```python
from build123d import *

# Parameters (mm, degrees)
SKETCH1_W           = 218
SKETCH1_H           = 465
BOSS_EXTRUDE1_DEPTH = 2
SKETCH2_W           = 30
SKETCH2_H           = 20
CUT_EXTRUDE1_DEPTH  = 8
BOSS_EXTRUDE2_DEPTH = 2


with BuildPart() as part:
    # Sketch1 → Boss-Extrude1 (new body)
    with BuildSketch(Plane.XY):
        Rectangle(SKETCH1_W, SKETCH1_H)
    extrude(amount=BOSS_EXTRUDE1_DEPTH)

    # Sketch2 → Cut-Extrude1 (cut)
    with BuildSketch(Plane.XY.offset(2)):
        Polygon((-61, 190), (-91, 190), (-91, 180), (-91, 170), (-61, 170), align=None)
        Polygon((-61, 145), (-91, 145), (-91, 135), (-91, 125), (-61, 125), align=None)
        with Locations((-76, 90)):
            Rectangle(SKETCH2_W, SKETCH2_H)
        with Locations((-76, 45)):
            Rectangle(SKETCH2_W, SKETCH2_H)
        with Locations((-76, 0)):
            Rectangle(SKETCH2_W, SKETCH2_H)
        with Locations((-76, -45)):
            Rectangle(SKETCH2_W, SKETCH2_H)
        with Locations((-76, -90)):
            Rectangle(SKETCH2_W, SKETCH2_H)
        with Locations((-76, -135)):
            Rectangle(SKETCH2_W, SKETCH2_H)
        with Locations((-76, -180)):
            Rectangle(SKETCH2_W, SKETCH2_H)
    extrude(amount=-CUT_EXTRUDE1_DEPTH, mode=Mode.SUBTRACT)

    # Sketch3 → Boss-Extrude2 (add)
    with BuildSketch(Plane.XY.offset(2)):
        Polygon((111, 164.5), (109, 164.5), (109, 139.5), (109, 114.5), (111, 114.5), align=None)
        Polygon((111, 71.5), (109, 71.5), (109, 46.5), (109, 21.5), (111, 21.5), align=None)
        Polygon((111, -114.5), (109, -114.5), (109, -139.5), (109, -164.5), (111, -164.5), align=None)
        Polygon((111, -21.5), (109, -21.5), (109, -46.5), (109, -71.5), (111, -71.5), align=None)
    extrude(amount=-BOSS_EXTRUDE2_DEPTH)


solid = part.part
```
Geometry check sheet. Reference: the model listing, model coordinates, mm. Coordinates: 2 decimals unless noted, no trailing zeros. Order: outer loops, then holes, each group sorted by start corner. A loop starts at its lowest first (then second) coordinate and runs counter-clockwise, first axis right, second up.
Item 1: Section check B-B (z = 1.65). Count the separate pieces of the cut face and the enclosed holes in it, plus the area to 3 significant figures.
Item 2: Section check A-A (y = -180). Enter the section's corners in (x, z), plus the area to 3 significant figures.
Item 3: Scan lines: line 1 along X through (y, z) = (-171, 0.7); line 2 along X through (y, z) = (-77, 0.95). Record each from-to range of solid material in increasing order.
Item 4: Depth check by flat-ended pin: pin 1 (0.6 mm diameter, centred on y = 0, z = 1, fed in from +X); pin 2 (1 mm diameter, centred on x = 110.5, z = 0.5, fed in from -Y); pin 3 (0.6 mm diameter, centred on x = 110, z = 0.5, fed in from +Y); pin 4 (1 mm diameter, centred on x = -26.5, y = 151, fed in from -Z). Enter the tip coordinate at first touch or a pass-through.
Check sheet entries:
1. separate pieces: 1
1. enclosed holes: 9
1. area: 96,400 mm2
2. outline: (-109, 0) - (-91, 0) - (-91, 2) - (-109, 2) - close; (-61, 0) - (109, 0) - (109, 2) - (-61, 2) - close
2. area: 376 mm2
3. line 1: x = -109 to -91, -61 to 109
3. line 2: x = -109 to 109
4. pin 1: stops at x = 109
4. pin 2: stops at y = -164.5
4. pin 3: stops at y = 164.5
4. pin 4: stops at z = 0
